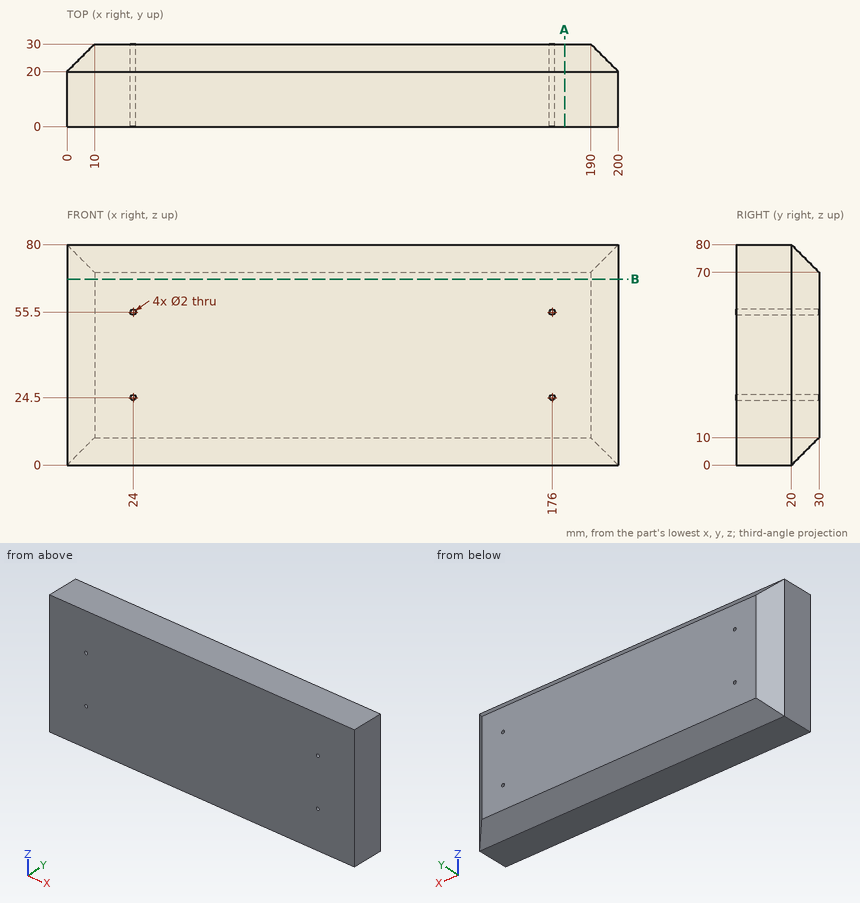
Input: dimensioned drawing with shaded views. Units: mm. Origin: part minimum x, y, z. Round coordinates to 2 decimals unless told otherwise and drop trailing zeros. Loops run counter-clockwise (first coordinate to the right, second up) from the corner with the lowest first, then second, coordinate; pieces in that order, holes last. Notation, with made-up numbers: M -36,-11 L -19,-11 A16 ccw -19,3 Z; hole C 2.25,80 d4. An arc over 180 degrees is marked long. Answer in a Markdown table with one row per item. Add a question column.
1. Ray query, probe 1 along X at (y, z) = (13.5, 55.5); probe 2 along Z at (x, y) = (24, 18.25); probe 3 along X at (y, z) = (21.75, 24.5). Return the intervals inside material, ascending.
2. Section A-A (x = 180.5). Output: boundary loops of the cut face in (y, z), and give its area (3 significant figures).
3. Contact query for flat-ended pins moving along their axis: pin 1 (3 mm diameter, centred on y = 24, z = 58.5, fed in from -X); pin 2 (1 mm diameter, centred on x = 124, y = 22.5, fed in from -Z). Output: stop coordinate, or through.
4. Section B-B (z = 67.5). Output: boundary loops of the cut face in (x, y).
Values follow:
| question | item | result |
|---|---|---|
| 1 | probe 1 | 0 to 23, 25 to 175, 177 to 200 |
| 1 | probe 2 | 0 to 23.5, 25.5 to 54.5, 56.5 to 80 |
| 1 | probe 3 | 1.75 to 23, 25 to 175, 177 to 198.25 |
| 2 | outline | M 0,0 L 20,0 L 30,10 L 30,70 L 20,80 L 0,80 Z |
| 2 | area | 2,300 mm^2 |
| 3 | pin 1 | x = 2.5 |
| 3 | pin 2 | z = 2 |
| 4 | outline | M 0,0 L 200,0 L 200,20 L 190,30 L 10,30 L 0,20 Z |
